```python
from build123d import *

# Parameters (mm, degrees)
SKETCH1_W           = 38.1
SKETCH1_H           = 31.75
SKETCH1_R           = 12.7
BOSS_EXTRUDE1_DEPTH = 2.38125
FILLET1_R           = 2.54


with BuildPart() as part:
    # Sketch1 → Boss-Extrude1 (new, symmetric)
    # profile 1 of 2: a face of its own
    with BuildSketch(Plane.XY):
        Polygon((-19.05, 6.35), (-19.05, 2.38125), (0, 2.38125), (0, -2.38125), (-19.05, -2.38125), (-19.05, -6.35), (19.05, -6.35), (19.05, 6.35), align=None)
    # profile 2 of 2: a face of its own
    with BuildSketch(Plane.XY):
        with Locations((0, 22.225)):
            Rectangle(SKETCH1_W, SKETCH1_H)
        with Locations(Location((0, 22.225, 0), (0, 0, 180))):
            Circle(SKETCH1_R, mode=Mode.SUBTRACT)
    extrude(amount=BOSS_EXTRUDE1_DEPTH, both=True)

    # Fillet1
    fillet1_edges = [part.edges().sort_by_distance(p)[0] for p in [
        (-19.05, 38.1, 0),
        (19.05, 38.1, 0),
        (19.05, -6.35, 0),
    ]]
    fillet(fillet1_edges, radius=FILLET1_R)


solid = part.part
```
Work out the finished part from the listing and answer in its coordinate system (mm). A direction names the side the tool comes from. Coordinates: 2 decimals unless noted, no trailing zeros. Write each loop counter-clockwise with the first axis right and the second up, starting at its lowest first coordinate (ties: lowest second). Pieces come first, ordered by that corner, then holes. Notation, with made-up numbers: (80.5, 23.5) - (111.5, 23.5) arc R29 ccw to (111.5, 50.5) - close; hole circle Ø2 at (52, 46). An arc over 180 degrees is marked (long way). Answer as a JSON object with one key per item and string values.
Q1. Find section B-B (x = 7). Write down the section's boundary in (y, z).
Results list:
{"outline": "(-6.35, -2.38) - (11.63, -2.38) - (11.63, 2.38) - (-6.35, 2.38) - close; (32.82, -2.38) - (38.1, -2.38) - (38.1, 2.38) - (32.82, 2.38) - close"}
Q2. Consider L1, parallel to Y at x = -6.5, z = 1.7; L2, parallel to X at y = 22, z = -0.1; L3, parallel to Y at x = -9, z = -0.6. Determine where each line is inside the solid, lowest interval first. Write a range as from..to.
Results list:
{"L1": "y = -6.35..-2.38, 2.38..11.31, 33.14..38.1", "L2": "x = -19.05..-12.7, 12.7..19.05", "L3": "y = -6.35..-2.38, 2.38..13.26, 31.19..38.1"}
Q3. Find section D-D (y = -1). Write down the section's boundary in (x, z).
Results list:
{"outline": "(0, -2.38) - (19.05, -2.38) - (19.05, 2.38) - (0, 2.38) - close"}
Q4. For a pull along Y with two mould halves and no side action, classify faces 1 (the cylindrical face through (18.326, -5.586, 0.033)), 2 (the flat face through (0, 6, 2.381)), 3 (the flat face through (-9, -2.381, 0)) as pulls with the +Y half, pulls with the -Y half, needs draft (parallel to the pull), parting line crosses it, or undercut.
Results list:
{"face 1": "pulls with the -Y half", "face 2": "needs draft", "face 3": "undercut"}
Q5. Which of the six approach directions +Z, -Z, +X, -X, +Y, -Y give full straight-line access (tool end or side, diameter ignored) to faces 4 (the flat face through (0, 0, 0)), 5 (the cylindrical face through (1.653, 9.633, -0.033))?
Results list:
{"face 4": "+Z, -Z, -X", "face 5": "+Z, -Z"}
Q6. Find section A-A (x = -3.5). Write down the section's boundary in (y, z).
Results list:
{"outline": "(-6.35, -2.38) - (-2.38, -2.38) - (-2.38, 2.38) - (-6.35, 2.38) - close; (2.38, -2.38) - (10.02, -2.38) - (10.02, 2.38) - (2.38, 2.38) - close; (34.43, -2.38) - (38.1, -2.38) - (38.1, 2.38) - (34.43, 2.38) - close"}
Q7. Given pin 1 Ø1.4 at (y, z) = (0.5, 0) entering from -X, flat-ended and moving along its own axis, determine where the tip first touches the part or whether it passes through.
Results list:
{"pin 1": "stops at x = 0"}
Q8. Find section C-C (z = 1.35). Write down the section's boundary in (x, y) (3 decimals).
Results list:
{"outline": "(-19.05, -6.35) - (16.51, -6.35) arc R2.54 ccw to (19.05, -3.81) - (19.05, 35.56) arc R2.54 ccw to (16.51, 38.1) - (-16.51, 38.1) arc R2.54 ccw to (-19.05, 35.56) - (-19.05, 2.381) - (0, 2.381) - (0, -2.381) - (-19.05, -2.381) - close; hole circle Ø25.4 at (0, 22.225)"}
